from build123d import *

# Parameters (mm, degrees)
SKETCH1_R                         = 69.723
BOSS_EXTRUDE1_DEPTH               = 41.656
SKETCH3_W                         = 5.588
SKETCH3_H                         = 9.652
SKETCH4_R                         = 66.167
BOSS_EXTRUDE2_DEPTH               = 19.8374
SKETCH5_W                         = 5.3975
SKETCH5_H                         = 7.1374
PIPE_TAP_DRILL_FOR_1_4_TAP1_D     = 11.1252
TAP_DRILL_FOR_3_8_16_TAP1_D       = 7.9375
TAP_DRILL_FOR_3_8_16_TAP1_DEPTH   = 25.4
TAP_DRILL_FOR_3_8_16_TAP1_TIP     = 2.384665582
PIPE_TAP_DRILL_FOR_1_4_TAP2_D     = 11.1252
PIPE_TAP_DRILL_FOR_1_4_TAP2_DEPTH = 61.4934
TAP_DRILL_FOR_3_8_16_TAP2_D       = 7.9375
TAP_DRILL_FOR_3_8_16_TAP2_DEPTH   = 19.05
TAP_DRILL_FOR_3_8_16_TAP2_TIP     = 2.384665582


with BuildPart() as part:
    # Sketch1 → Boss-Extrude1 (new body)
    with BuildSketch(Plane(origin=(0, 0, 0), x_dir=(1, 0, 0), z_dir=(0, 1, 0))):
        with Locations(Location((0, 0, 0), (0, 0, 270))):
            Circle(SKETCH1_R)
    extrude(amount=BOSS_EXTRUDE1_DEPTH)

    # Sketch3 → Cut-Revolve1 (revolve, cut)
    with BuildSketch(Plane(origin=(0, 0, 0), x_dir=(0, 0, -1), z_dir=(1, 0, 0)), mode=Mode.PRIVATE) as cut_revolve1_sk:
        with Locations((66.929, 27.178)):
            Rectangle(SKETCH3_W, SKETCH3_H)
        with Locations((66.929, 11.176)):
            Rectangle(SKETCH3_W, SKETCH3_H)
    revolve(cut_revolve1_sk.sketch.rotate(Axis((0, 41.656, 0), (0, -1, 0)), 180), axis=Axis((0, 41.656, 0), (0, -1, 0)), mode=Mode.SUBTRACT)

    # Sketch4 → Boss-Extrude2 (add)
    with BuildSketch(Plane.XZ):
        with Locations(Location((0, 0, 0), (0, 0, 270))):
            Circle(SKETCH4_R)
    extrude(amount=BOSS_EXTRUDE2_DEPTH)

    # Sketch5 → Cut-Revolve2 (revolve, cut)
    with BuildSketch(Plane(origin=(0, 0, 0), x_dir=(0, 0, -1), z_dir=(1, 0, 0)), mode=Mode.PRIVATE) as cut_revolve2_sk:
        with Locations((63.46825, -9.9187)):
            Rectangle(SKETCH5_W, SKETCH5_H)
    revolve(cut_revolve2_sk.sketch.rotate(Axis((0, 41.656, 0), (0, -1, 0)), 180), axis=Axis((0, 41.656, 0), (0, -1, 0)), mode=Mode.SUBTRACT)

    # Pipe Tap Drill for 1/4 Tap1 (through all)
    with Locations(Plane(origin=(0, 41.656, -38.1), x_dir=(0, 0, 1), z_dir=(0, 1, 0))):
        with Locations((0, 0)):
            pipe_tap_drill_for_1_4_tap1 = Hole(PIPE_TAP_DRILL_FOR_1_4_TAP1_D / 2)

    # Mirror1: Pipe Tap Drill for 1/4 Tap1 across plane
    add(pipe_tap_drill_for_1_4_tap1.mirror(Plane.XY), mode=Mode.SUBTRACT)

    # Tap Drill for 3/8-16 Tap1
    with Locations(Plane.ZX.offset(41.656)):
        with Locations((0, 0)):
            Hole(TAP_DRILL_FOR_3_8_16_TAP1_D / 2, depth=TAP_DRILL_FOR_3_8_16_TAP1_DEPTH)
            with Locations((0, 0, -(TAP_DRILL_FOR_3_8_16_TAP1_DEPTH + TAP_DRILL_FOR_3_8_16_TAP1_TIP / 2))):  # 118° drill point
                Cone(0, TAP_DRILL_FOR_3_8_16_TAP1_D / 2, TAP_DRILL_FOR_3_8_16_TAP1_TIP, mode=Mode.SUBTRACT)

    # Pipe Tap Drill for 1/4 Tap2
    with Locations(Plane(origin=(0, 41.656, 38.1), x_dir=(0, 0, 1), z_dir=(0, 1, 0))):
        with Locations((0, 0), (-76.2, 0)):
            Hole(PIPE_TAP_DRILL_FOR_1_4_TAP2_D / 2, depth=PIPE_TAP_DRILL_FOR_1_4_TAP2_DEPTH)

    # Tap Drill for 3/8-16 Tap2
    with Locations(Plane(origin=(-44.45, 41.656, 0), x_dir=(0, 0, 1), z_dir=(0, 1, 0))):
        with Locations((0, 0), (0, 88.9)):
            Hole(TAP_DRILL_FOR_3_8_16_TAP2_D / 2, depth=TAP_DRILL_FOR_3_8_16_TAP2_DEPTH)
            with Locations((0, 0, -(TAP_DRILL_FOR_3_8_16_TAP2_DEPTH + TAP_DRILL_FOR_3_8_16_TAP2_TIP / 2))):  # 118° drill point
                Cone(0, TAP_DRILL_FOR_3_8_16_TAP2_D / 2, TAP_DRILL_FOR_3_8_16_TAP2_TIP, mode=Mode.SUBTRACT)


solid = part.part
Geometry: final body of the model. Coordinates: model frame, mm. A direction names the side the tool comes from. Coordinates: 2 decimals unless noted, no trailing zeros. Loops run counter-clockwise (first coordinate to the right, second up) from the corner with the lowest first, then second, coordinate; pieces in that order, holes last. Notation, with made-up numbers: (69.25, 79.5) - (73.25, 79.5) arc R11 cw to (73.25, 94.5) - close; hole circle Ø5 at (-23.75, 26.25). An arc over 180 degrees is marked (long way). One line per question, with ' | ' between items. Start each with the question number.
(1) Cut plane A-A on y = 4. Output: boundary loops of the cut face in (x, z), and give its area (3 significant figures).
(2) Ray query, L1, parallel to X at y = 32.5, z = 0; L2, parallel to Y at x = 43, z = 52; L3, parallel to Y at x = 59, z = -27. Return the intervals inside material, ascending. Write a range as from..to.
(3) First-contact query: pin 1 (7 mm diameter, centred on x = 0, z = 0, fed in from +Y); pin 2 (1 mm diameter, centred on x = 25, y = 6, fed in from -Z); pin 3 (4 mm diameter, centred on x = -31, y = 13, fed in from +Z); pin 4 (18 mm diameter, centred on x = 0, z = 38.1, fed in from +Y). Flat tips, straight axial feed; report the tip coordinate or a pass-through.
(4) Draft query along X for faces 4 (the cylindrical face through (48.385, 31.998, 0.517)), 5 (the cylindrical face through (-19.264, 11.244, 61.173)), 6 (the conical face through (-43.767, 20.635, -0.09)), 7 (the flat face through (-62, 0, 25)). Return one class per face: +X half, -X half, draft (parallel to the pull), parting line (faces both ways), or undercut.
(5) Reachability of faces 1 (the flat face through (56.5, 6.35, -30.7)), 2 (the cylindrical face through (-40.26, -16.62, 52.51)), 3 (the cylindrical face through (-3.874, 28.778, 0.86)) from +Z, -Z, +X, -X, +Y, -Y: full face, straight path, thin tool, end or side. Return the list, or none.
Here are the results:
1) outline: circle Ø139.45 at (0, 0); hole circle Ø11.13 at (0, -38.1); hole circle Ø11.13 at (0, 38.1) | area: 15,100 mm²
2) L1: -69.72..-48.42, -40.48..-3.97, 3.97..40.48, 48.42..69.72 | L2: 0..6.35, 16..22.35, 32..41.66 | L3: -19.84..-13.49, -6.35..6.35, 16..22.35, 32..41.66
3) pin 1: y = 15.97 | pin 2: z = -65.28 | pin 3: z = 57.2 | pin 4: y = 41.66
4) face 4: undercut | face 5: parting line | face 6: undercut | face 7: draft
5) face 1: none | face 2: -Y | face 3: +Y
